Could you check a few things on this model? Use its own coordinates, in mm. Face numbers are marked on the shaded views. Round coordinates to 2 decimals unless told otherwise and drop trailing zeros. Loops run counter-clockwise (first coordinate to the right, second up) from the corner with the lowest first, then second, coordinate; pieces in that order, holes last. Notation, with made-up numbers: (30, -4) -> (66, -4) arc R20 cw to (66, 24) -> close; hole circle Ø10 at (-7.75, 23). An arc over 180 degrees is marked (long way). One line per item, written item: value.
```python
from build123d import *

# Parameters (mm, degrees)
BOSS_EXTRUDE1_DEPTH = 170
SKETCH3_R           = 1.5
CUT_EXTRUDE2_DEPTH  = 170
SKETCH4_R           = 1.3
CUT_EXTRUDE3_DEPTH  = 200


with BuildPart() as part:
    # Sketch2 → Boss-Extrude1 (new body)
    with BuildSketch(Plane(origin=(0, 0, 0), x_dir=(0, 0, -1), z_dir=(1, 0, 0))):
        with BuildLine():
            Line((-80, 0), (80, 0))
            ThreePointArc((80, 0), (85.303300859, 2.196699141), (87.5, 7.5))
            Line((87.5, 7.5), (87.5, 20))
            Line((87.5, 20), (85.5, 20))
            Line((85.5, 20), (85.5, 7))
            ThreePointArc((85.5, 7), (84.035533906, 3.464466094), (80.5, 2))
            Line((80.5, 2), (-80.5, 2))
            ThreePointArc((-80.5, 2), (-84.035533906, 3.464466094), (-85.5, 7))
            Line((-85.5, 7), (-85.5, 20))
            Line((-85.5, 20), (-87.5, 20))
            Line((-87.5, 20), (-87.5, 7.5))
            ThreePointArc((-87.5, 7.5), (-85.303300859, 2.196699141), (-80, 0))
        make_face()
    extrude(amount=BOSS_EXTRUDE1_DEPTH)

    # Sketch3 → Cut-Extrude2 (cut)
    with BuildSketch(Plane(origin=(0, 2, 0), x_dir=(1, 0, 0), z_dir=(0, 1, 0))):
        with Locations(Location((20, -5.5, 0), (0, 0, 270))):
            Circle(SKETCH3_R)
        with Locations(Location((150, -5.5, 0), (0, 0, 270))):
            Circle(SKETCH3_R)
    extrude(amount=-CUT_EXTRUDE2_DEPTH, mode=Mode.SUBTRACT)

    # Sketch4 → Cut-Extrude3 (cut)
    with BuildSketch(Plane.XY.offset(87.5)):
        with Locations((90, 14)):
            Circle(SKETCH4_R)
    extrude(amount=-CUT_EXTRUDE3_DEPTH, mode=Mode.SUBTRACT)


solid = part.part
```
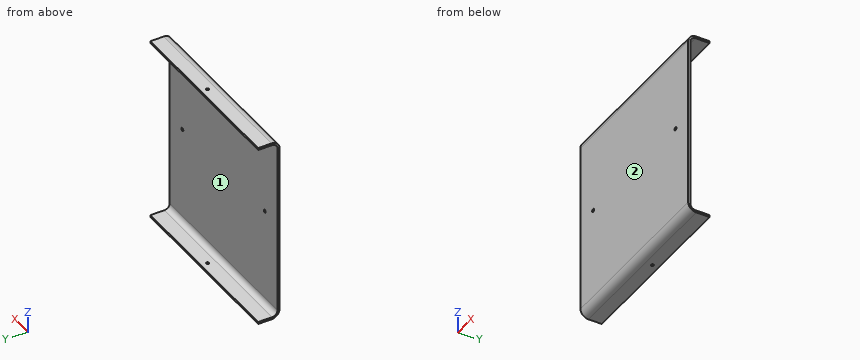
Item 1: If we mould it in two halves opening along Z, with no side actions, what happens to the marked faces 1 and 2? For each: released by +Z, released by -Z, zero draft, split by the parting line, or undercut.
Output:
face 1: undercut
face 2: zero draft
Item 2: If we section it at C-C on z = -46.5: List the corners of the cut face in (x, y) for me, plus the area to 3 significant figures.
Output:
outline: (0, 0) -> (170, 0) -> (170, 2) -> (0, 2) -> close
area: 340 mm²
Item 3: Will these pins go through, and if not, where does the flat tip stop? pin 1 Ø1.5 at (x, z) = (114.5, -0.5) entering from +Y; pin 2 Ø2.5 at (x, z) = (150, 5.5) entering from +Y.
Output:
pin 1: stops at y = 2
pin 2: passes through
Item 4: If we section it at A-A on y = 17.5: List the corners of the cut face in (x, z) for me.
Output:
outline: (0, -87.5) -> (170, -87.5) -> (170, -85.5) -> (0, -85.5) -> close; (0, 85.5) -> (170, 85.5) -> (170, 87.5) -> (0, 87.5) -> close
Item 5: If we section it at B-B on x = 27.5: List the corners of the cut face in (y, z) for me.
Output:
outline: (0, -80) arc R7.5 ccw to (7.5, -87.5) -> (20, -87.5) -> (20, -85.5) -> (7, -85.5) arc R5 cw to (2, -80.5) -> (2, 80.5) arc R5 cw to (7, 85.5) -> (20, 85.5) -> (20, 87.5) -> (7.5, 87.5) arc R7.5 ccw to (0, 80) -> close
Item 6: I need wall thicknesses on line 1 (Z direction, x = 105.5, y = 18.5); line 2 (Y direction, x = 103, z = -54); line 3 (Z direction, x = 150, y = 1.55). Which ranges of each line are inside material? Lowest first, please. Write a range as from..to.
Output:
line 1: z = -87.5..-85.5, 85.5..87.5
line 2: y = 0..2
line 3: z = -84.57..4, 7..84.57
